Check sheet for the modelled part. Datum: model origin and axes. Units: mm. A direction names the side the tool comes from. Coordinates: 2 decimals unless noted, no trailing zeros. Loops run counter-clockwise (first coordinate to the right, second up) from the corner with the lowest first, then second, coordinate; pieces in that order, holes last. Notation, with made-up numbers: M 19.25,-19 L 30.25,-19 A25 ccw 30.25,14 Z; hole C 74.25,-21 d9. An arc over 180 degrees is marked long. Use CSV: the item, a comma, the result in double quotes. Start each with the question number.
(1) Go/stop test with flat-tipped pins: pin 1 Ø6 at (x, z) = (-12.5, 44) entering from +Y; pin 2 Ø7 at (y, z) = (-23, 50.5) entering from +X; pin 3 Ø2.5 at (x, z) = (-3.5, 72.5) entering from +Y. Record where each tip stops, or that it passes through.
(2) Section check B-B on z = 58. Record the cut outline in (x, y).
(3) Section check A-A on y = 0. Record the cut outline in (x, z), and give its area (3 significant figures).
(4) Set-up check for faces 1 (the flat face through (5, 15, 49)), 2 (the flat face through (0, -22, 49)), 3 (the cylindrical face through (-24.994, 0.55, 46.342)), 4 (the flat face through (0, 21, 49)), 5 (the flat face through (-5, -15, 49)): record each of +Z, -Z, +X, -X, +Y, -Y from which the full face is reachable in a straight line by a thin tool's end or side.
(5) Draft check along Y on faces 6 (the flat face through (-14, 0, 0)), 7 (the flat face through (3, 17.5, 49)), 8 (the flat face through (-2, -18.75, 49)). Enter one of: pulls with the +Y half, pulls with the -Y half, needs draft (parallel to the pull), parting line crosses it, or undercut.
(6) Scan lines: line 1 (Y direction, x = -6, z = 6); line 2 (Y direction, x = 2.5, z = 26.5); line 3 (Y direction, x = -1, z = 41). Record each from-to range of solid material in increasing order.
from build123d import *

# Parameters (mm, degrees)
F1_DEPTH    = 100
F2_T2_ANGLE = 248.8655063523


# Not quite as in the source:
# - a fillet or chamfer that OpenCascade refuses, or shapes differently, is made with other operations: its cross-section is extruded or revolved along the edge and cut away or added


with BuildPart() as f1:
    # F0 (on Top) → F1 (new body)
    with BuildSketch(Plane.XY):
        with BuildLine():
            ThreePointArc((-5, -11.4564392374), (-12.2363289116, 2.5538705461), (0, 12.5))
            Line((0, 12.5), (5, 12.5))
            Line((5, 12.5), (5, 17.5))
            Line((5, 17.5), (0, 17.5))
            Line((0, 17.5), (0, 25))
            ThreePointArc((0, 25), (-25, 0), (0, -25))
            Line((0, -25), (0, -18.75))
            Line((0, -18.75), (-5, -18.75))
            Line((-5, -18.75), (-5, -11.4564392374))
        make_face()
    extrude(amount=F1_DEPTH)

    # F2: fillet of radius 6 on 1 edges, made by hand

    # F2_s1 → F2_t2 (revolve, cut)
    with BuildSketch(Plane(origin=(0, 0, 0), x_dir=(0, 0, 1), z_dir=(0.8247903997, -0.5654385878, 0))):
        with BuildLine():
            ThreePointArc((94, -25), (98.2426406871, -23.2426406871), (100, -19))
            Line((100, -19), (100, -25))
            Line((100, -25), (94, -25))
        make_face()
    revolve(axis=Axis((0, 0, 100), (0, 0, 1)), revolution_arc=F2_T2_ANGLE, mode=Mode.SUBTRACT)


solid = f1.part
Outcome:
1,pin 1,"stops at y = 23.12"
1,pin 2,"stops at x = 0"
1,pin 3,"stops at y = 24.9"
2,outline,"M -5,-18.75 L -5,-11.46 A12.5 cw 0,12.5 L 5,12.5 L 5,17.5 L 0,17.5 L 0,25 A25 ccw 0,-25 L 0,-18.75 Z"
3,outline,"M -25,0 L -12.5,0 L -12.5,100 L -19,100 A6 ccw -25,94 Z"
3,area,"1,240 mm²"
4,face 1,"+Z, -Z, +X, +Y, -Y"
4,face 2,"+Z, -Z, +X, -Y"
4,face 3,"+Z, -Z, -X"
4,face 4,"+Z, -Z, +X, +Y"
4,face 5,"+Z, -Z, +X"
5,face 6,"needs draft"
5,face 7,"pulls with the +Y half"
5,face 8,"undercut"
6,line 1,"y = -24.27 to -10.97, 10.97 to 24.27"
6,line 2,"y = 12.5 to 17.5"
6,line 3,"y = -24.98 to -18.75, 12.46 to 24.98"
